```python
from build123d import *

# Parameters (mm, degrees)
F1_DEPTH = 25.4
F2_W     = 25.4
F2_H     = 114.3
F3_DEPTH = 127
F4_W     = 25.4
F4_H     = 114.3
F5_DEPTH = 127
F6_W     = 19.05
F6_H     = 19.05
F7_DEPTH = 25.401


with BuildPart() as f1:
    # F0 (on Front) → F1 (new body)
    with BuildSketch(Plane.XZ):
        with BuildLine():
            Line((635, -76.2), (635, 76.2))
            Line((635, 76.2), (-635, 76.2))
            Line((-635, 76.2), (-635, -76.2))
            ThreePointArc((-635, -76.2), (0, -31.75), (635, -76.2))
        make_face()
    extrude(amount=F1_DEPTH)

    # F2 (on face) → F3 (join)
    with BuildSketch(Plane(origin=(-635, 0, 0), x_dir=(0, -1, 0), z_dir=(-1, 0, 0))):
        with Locations((12.7, 0)):
            Rectangle(F2_W, F2_H)
    extrude(amount=F3_DEPTH)

    # F4 (on face) → F5 (join)
    with BuildSketch(Plane.YZ.offset(635)):
        with Locations((-12.7, 0)):
            Rectangle(F4_W, F4_H)
    extrude(amount=F5_DEPTH)

    # F6 (on face) → F7 (cut, through all)
    with BuildSketch(Plane.XZ.offset(25.4)):
        with Locations((-719.1375, 0)):
            Rectangle(F6_W, F6_H)
        with Locations((719.1375, 0)):
            Rectangle(F6_W, F6_H)
    extrude(amount=-F7_DEPTH, mode=Mode.SUBTRACT)


solid = f1.part
```
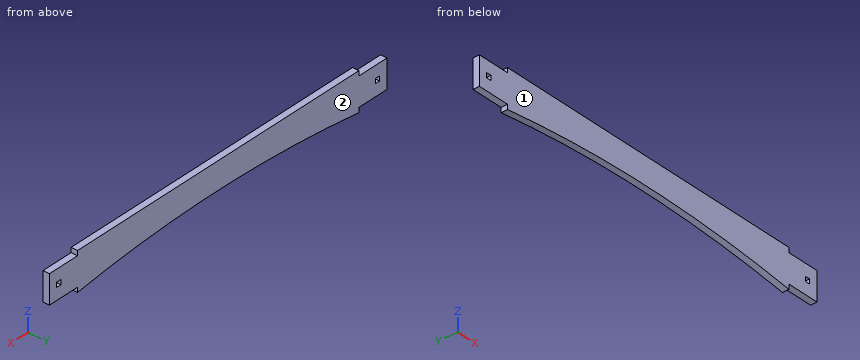
Design review of the part built by this model. Coordinates are the model's own, in mm. Face numbers are marked on the shaded views. Give positions to 0.01 mm unless a question says otherwise; leave off trailing zeros. Order: outer loops, then holes, each group sorted by start corner. A loop starts at its lowest first (then second) coordinate and runs counter-clockwise, first axis right, second up. Notation, with made-up numbers: M 69,30.5 L 81,30.5 A26 ccw 81,57.5 Z; hole C -29,36.25 d1. An arc over 180 degrees is marked long. One line per question, with ' | ' between items. Start each with the question number.
Q1. For pin 1 Ø9.5 at (x, y) = (-716.5, -15.5) entering from +Z; pin 2 Ø5 at (x, z) = (430, 40) entering from +Y; pin 3 Ø9.5 at (y, z) = (-6.5, 70.5) entering from +X; pin 4 Ø9.5 at (x, y) = (-719, -13) entering from -Z, all flat-tipped, find the tip position at first contact; note any pin that passes through.
Q2. For L1, parallel to X at y = -5, z = -2.5; L2, parallel to Z at x = 690.5, y = -22.75; L3, parallel to X at y = -19.25, z = 60, list the stretches that pass through material, from the lowest coordinate up. Write a range as [from, to].
Q3. We need section C-C (x = 253). Write out the cut boundary in (y, z), plus the area to 3 significant figures.
Q4. The part is to be moulded in two halves that separate along Y. For the marked faces 1 and 2, say which applies: +Y half, -Y half, draft (parallel to the pull), parting line (faces both ways), or undercut.
Q5. We need section A-A (y = -10.5). State how many separate pieces and enclosed holes the cut face has, plus the area to 3 significant figures.
Q6. We need section B-B (x = -221). Write out the cut boundary in (y, z), plus the area to 3 significant figures.
Returned:
1) pin 1: z = 57.15 | pin 2: y = 0 | pin 3: x = 635 | pin 4: z = -57.15
2) L1: [-762, -728.66], [-709.61, 709.61], [728.66, 762] | L2: [-57.15, 57.15] | L3: [-635, 635]
3) outline: M -25.4,-38.78 L 0,-38.78 L 0,76.2 L -25.4,76.2 Z | area: 2,920 mm2
4) face 1: -Y half | face 2: +Y half
5) separate pieces: 1 | enclosed holes: 2 | area: 184,000 mm2
6) outline: M -25.4,-37.11 L 0,-37.11 L 0,76.2 L -25.4,76.2 Z | area: 2,880 mm2
